Can you work these out from the model? Positions are in its coordinate system, mm. Face numbers are marked on the shaded views. A direction names the side the tool comes from. Round coordinates to 2 decimals unless told otherwise and drop trailing zeros. Write each loop counter-clockwise with the first axis right and the second up, starting at its lowest first coordinate (ties: lowest second). Pieces come first, ordered by that corner, then holes. Notation, with made-up numbers: (43, 38.25) -> (90, 38.25) arc R18 ccw to (90, 72.25) -> close; hole circle Ø3 at (-40, 81.5). An arc over 180 degrees is marked (long way). Use CSV: the item, a comma, the result in double quotes.
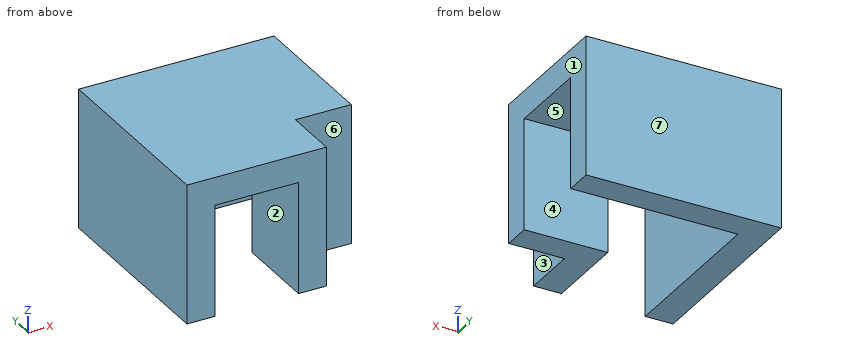
```python
from build123d import *

# Parameters (mm, degrees)
BOSS_EXTRU_1_DEPTH      = 5
ESQUISSE2_W             = 3
ESQUISSE2_H             = 4
ENL_V_MAT_EXTRU_1_DEPTH = 6
ESQUISSE3_W             = 4
ESQUISSE3_H             = 3
ENL_V_MAT_EXTRU_2_DEPTH = 6


with BuildPart() as part:
    # Esquisse1 → Boss.-Extru.1 (new body)
    with BuildSketch(Plane.XY):
        Polygon((-1.317889251, -4.63356974), (-1.317889251, -2.63356974), (0.682110749, -2.63356974), (0.682110749, 2.36643026), (-6.317889251, 2.36643026), (-6.317889251, -4.63356974), align=None)
    extrude(amount=BOSS_EXTRU_1_DEPTH)

    # Esquisse2 → Enlèv. mat.-Extru.1 (cut)
    with BuildSketch(Plane.XZ.offset(4.63356974)):
        with Locations((-3.817889251, 2)):
            Rectangle(ESQUISSE2_W, ESQUISSE2_H)
    extrude(amount=-ENL_V_MAT_EXTRU_1_DEPTH, mode=Mode.SUBTRACT)

    # Esquisse3 → Enlèv. mat.-Extru.2 (cut)
    with BuildSketch(Plane(origin=(0.682110749, 0, 0), x_dir=(0, 0, -1), z_dir=(1, 0, 0))):
        with Locations((-2, -0.13356974)):
            Rectangle(ESQUISSE3_W, ESQUISSE3_H)
    extrude(amount=-ENL_V_MAT_EXTRU_2_DEPTH, mode=Mode.SUBTRACT)


solid = part.part
```
Q1. Please list where these lines run through material, in increasing order: probe 1 along X at (y, z) = (-3.5, 0.35); probe 2 along Y at (x, z) = (-2, 3.4); probe 3 along Y at (x, z) = (0, 0.85).
Resolved:
probe 1,"x = -6.32 to -5.32, -2.32 to -1.32"
probe 2,"y = -4.63 to -1.63, 1.37 to 2.37"
probe 3,"y = -2.63 to -1.63, 1.37 to 2.37"
Q2. If we mould it in two halves opening along Y, with no side actions, what happens to the marked faces 4, 5, 6 and 7? For each: released by +Y, released by -Y, zero draft, split by the parting line, or undercut.
Resolved:
face 4,"undercut"
face 5,"undercut"
face 6,"released by -Y"
face 7,"released by +Y"
Q3. Suppose I cut it at C-C (y = -2.25). Write out the boundary of the cut face in (x, z), and give its area (3 significant figures).
Resolved:
outline,"(-6.32, 0) -> (-5.32, 0) -> (-5.32, 4) -> (-2.32, 4) -> (-2.32, 0) -> (0.68, 0) -> (0.68, 5) -> (-6.32, 5) -> close"
area,"23.0 mm^2"
Q4. Will this pin go through, and if not, where does the flat tip stop? P1, Ø1, axis at x = -0.5, z = 2.5, coming from the -Y side.
Resolved:
P1,"stops at y = -2.63"
Q5. Suppose I cut it at A-A (z = 2.1). Write out the boundary of the cut face in (x, y), and give its area (3 significant figures).
Resolved:
outline,"(-6.32, -4.63) -> (-5.32, -4.63) -> (-5.32, 1.37) -> (0.68, 1.37) -> (0.68, 2.37) -> (-6.32, 2.37) -> close; (-2.32, -4.63) -> (-1.32, -4.63) -> (-1.32, -2.63) -> (0.68, -2.63) -> (0.68, -1.63) -> (-2.32, -1.63) -> close"
area,"18.0 mm^2"
Q6. On a 3-axis mill with a long thin cutter (end or side, diameter ignored), from which of +Z, -Z, +X, -X, +Y, -Y can I reach the whole of each face in a straight line? I mean the marked faces 1, 2 and 3. Say none if no direction works.
Resolved:
face 1,"+Z, -Z, +X, +Y, -Y"
face 2,"-Z, -Y"
face 3,"+Z, -Z, +X, -Y"
Q7. Suppose I cut it at D-D (x = -4.25). Write out the boundary of the cut face in (y, z), and give its area (3 significant figures).
Resolved:
outline,"(-4.63, 4) -> (1.37, 4) -> (1.37, 0) -> (2.37, 0) -> (2.37, 5) -> (-4.63, 5) -> close"
area,"11.0 mm^2"
Q8. Suppose I cut it at B-B (x = 0). Write out the boundary of the cut face in (y, z).
Resolved:
outline,"(-2.63, 0) -> (-1.63, 0) -> (-1.63, 4) -> (1.37, 4) -> (1.37, 0) -> (2.37, 0) -> (2.37, 5) -> (-2.63, 5) -> close"
